```python
from build123d import *

# Parameters (mm, degrees)
BOSS_EXTRUDE1_DEPTH = 38.1
BOSS_EXTRUDE2_START = 10.16
SKETCH2_R           = 3.175
BOSS_EXTRUDE2_DEPTH = 10.16


with BuildPart() as part:
    # Sketch1 → Boss-Extrude1 (new body)
    with BuildSketch(Plane(origin=(0, 0, 0), x_dir=(1, 0, 0), z_dir=(0, 1, 0))):
        with BuildLine():
            Line((-3.174725922, 0.04171715), (-1.172129839, 152.44171715))
            ThreePointArc((-1.172129839, 152.44171715), (2.044313233, 155.574725922), (5.177322005, 152.35828285))
            Line((5.177322005, 152.35828285), (3.174725922, -0.04171715))
            ThreePointArc((3.174725922, -0.04171715), (-0.04171715, -3.174725922), (-3.174725922, 0.04171715))
        make_face()
    extrude(amount=BOSS_EXTRUDE1_DEPTH)

    # Sketch2 → Boss-Extrude2 (add)
    with BuildSketch(Plane(origin=(0, 0, 0), x_dir=(-1, 0, 0), z_dir=(0, -1, 0)).offset(BOSS_EXTRUDE2_START)):
        with Locations(Location((-2.002596083, 152.4, 0), (0, 0, 90))):
            Circle(SKETCH2_R)
        with Locations(Location((0, 0, 0), (0, 0, 90))):
            Circle(SKETCH2_R)
    extrude(amount=-BOSS_EXTRUDE2_DEPTH)


solid = part.part
```
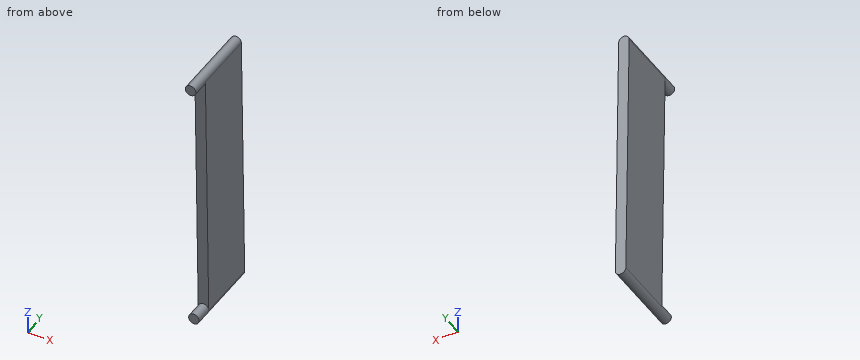
Source: CAD feature listing. Evaluate the final solid. Frame: model axes, mm. Coordinates: 2 decimals unless noted, no trailing zeros. Write each loop counter-clockwise with the first axis right and the second up, starting at its lowest first coordinate (ties: lowest second). Pieces come first, ordered by that corner, then holes. Notation, with made-up numbers: (61.5, 34) -> (99.5, 34) arc R19 cw to (99.5, 54) -> close; hole circle Ø10 at (68.25, -20). An arc over 180 degrees is marked (long way). Return JSON: item names as keys, results as strings. Group by question number.
1) Contact query for flat-ended pins moving along their axis: P1, Ø6, axis at y = 11, z = -99, coming from the -X side; P2, Ø1.5, axis at x = 3, z = -48.5, coming from the -Y side; P3, Ø6, axis at y = 18, z = -39, coming from the +X side. Output: stop coordinate, or through.
2) Section query A-A, the plane z = -57. Return loops of the section in (x, y).
3) Ray query, line 1 along Y through (x, z) = (3.5, -112.5); line 2 along X through (y, z) = (31.5, -130.5); line 3 along X through (y, z) = (21, -15). Return the intervals inside material, ascending.
From the geometry:
{
 "1": {"P1": "x = -1.91", "P2": "y = 0", "P3": "x = 3.73"},
 "2": {"outline": "(-2.43, 0) -> (3.92, 0) -> (3.92, 38.1) -> (-2.43, 38.1) -> close"},
 "3": {"line 1": "0 to 38.1", "line 2": "-1.46 to 4.89", "line 3": "-2.98 to 3.37"}
}
